```python
from build123d import *

# Parameters (mm, degrees)
CUT_EXTRUDE1_DEPTH = 4.7625
SKETCH6_R          = 2.749630657
CUT_EXTRUDE4_DEPTH = 4.7625
CUT_EXTRUDE4_DRAFT = -45


with BuildPart() as part:
    # Sketch4 → Revolve1 (revolve)
    with BuildSketch(Plane(origin=(0, 0, 0), x_dir=(0, 0, -1), z_dir=(1, 0, 0))):
        Polygon((-28.575, 7.14375), (-34.210625, 7.14375), (-34.925, 6.429375), (-34.925, 0), (22.225, 0), (22.225, 4.500033333), (21.962533333, 4.7625), (-26.2128, 4.7625), (-26.450925, 4.524375), (-28.336875, 4.524375), (-28.575, 4.7625), align=None)
    revolve(axis=Axis((0, 0, 34.925), (0, 0, -1)))

    # Sketch5 → Cut-Extrude1 (cut)
    with BuildSketch(Plane.XY.offset(34.925)):
        Polygon((2.38125, 1.374815329), (0, 2.749630657), (-2.38125, 1.374815329), (-2.38125, -1.374815329), (0, -2.749630657), (2.38125, -1.374815329), align=None)
    extrude(amount=-CUT_EXTRUDE1_DEPTH, mode=Mode.SUBTRACT)


with BuildPart() as cut_extrude4_tool:
    # Sketch6 → Cut-Extrude4 (with draft: the straight prism first)
    with BuildSketch(Plane.XY.offset(34.925)):
        Circle(SKETCH6_R)
    extrude(amount=-CUT_EXTRUDE4_DEPTH)
    # Cut-Extrude4: the draft: its side faces are tilted about the plane it starts from
    cut_extrude4_sides = [cut_extrude4_tool.faces().sort_by_distance(p)[0] for p in [
        (-2.749630657, 0, 32.54375),
    ]]
    draft(cut_extrude4_sides, Plane.XY.offset(34.925), CUT_EXTRUDE4_DRAFT)


with BuildPart() as part_1:
    add(part.part)

    # Cut-Extrude4: cut by cut_extrude4_tool
    add(cut_extrude4_tool.part, mode=Mode.SUBTRACT)

    # Sketch7 → Revolve2 (revolve)
    with BuildSketch(Plane(origin=(0, 0, 0), x_dir=(0, 0, -1), z_dir=(1, 0, 0))):
        Polygon((22.225, 3.9751), (33.866666667, 3.9751), (34.925, 2.916766667), (34.925, 0), (22.225, 0), align=None)
    revolve(axis=Axis((0, 0, -34.925), (0, 0, 1)))

    # Sketch10 → Cut-Revolve1 (revolve, cut)
    with BuildSketch(Plane(origin=(0, 0, 0), x_dir=(0, 0, -1), z_dir=(1, 0, 0))):
        with BuildLine():
            Line((23.1902, 3.0099), (25.0444, 3.0099))
            Line((25.0444, 3.0099), (26.797, 4.7625))
            Line((26.797, 4.7625), (22.225, 4.7625))
            Line((22.225, 4.7625), (22.225, 3.9751))
            ThreePointArc((22.225, 3.9751), (22.507700535, 3.292600535), (23.1902, 3.0099))
        make_face()
    revolve(axis=Axis((0, 0, -34.925), (0, 0, 1)), mode=Mode.SUBTRACT)


solid = part_1.part
```
Work out the finished part from the listing and answer in its coordinate system (mm). A direction names the side the tool comes from. Give positions to 0.01 mm unless a question says otherwise; leave off trailing zeros. Write each loop counter-clockwise with the first axis right and the second up, starting at its lowest first coordinate (ties: lowest second). Pieces come first, ordered by that corner, then holes.
(1) The part is cut by section A-A on z = -5.5. Write down the section's boundary in (x, y) (1 decimal), plus the area to 3 significant figures.
Final values:
outline: circle Ø9.5 at (0, 0)
area: 71.3 mm2
(2) Flat-ended cylindrical pins translate along their axes: pin 1 Ø3 at (x, z) = (-5.5, 23.5) entering from +Y; pin 2 Ø4 at (x, z) = (1.5, 16.5) entering from +Y; pin 3 Ø6 at (x, y) = (5, 4) entering from -Z. Find the tip coordinate at first contact, or state that the pin passes through.
Final values:
pin 1: stops at y = 2.58
pin 2: stops at y = 4.76
pin 3: stops at z = -34.44
(3) The mould has two halves that part along X. Classify faces 1 (the cylindrical face through (-2.9, -3.78, 2.46)), 2 (the flat face through (0, 3, 34.925)), 3 (the conical face through (1.27, -2.23, 34.74)), 4 (the flat face through (-1.174, 2.072, 32.577)): pulls with the +X half, pulls with the -X half, needs draft (parallel to the pull), parting line crosses it, or undercut.
Final values:
face 1: parting line crosses it
face 2: needs draft
face 3: undercut
face 4: undercut
(4) Straight lines are drawn through the part: line 1 (Z direction, x = 4.25, y = 2.5) (3 decimals); line 2 (Z direction, x = -3.25, y = -3) (3 decimals); line 3 (X direction, y = 1, z = -15). For each, find the intervals that lie inside material, in ascending order.
Final values:
line 1: z = 28.575 to 34.925
line 2: z = -22.225 to 34.925
line 3: x = -4.66 to 4.66
(5) Which of the six approach directions +Z, -Z, +X, -X, +Y, -Y give full straight-line access (tool end or side, diameter ignored) to faces 5 (the cylindrical face through (0.314, -7.137, 31.432)), 6 (the flat face through (-3, -3, -22.225)), 7 (the flat face through (0, 0, 30.162)), 8 (the cylindrical face through (-2.753, -3.59, 27.407))?
Final values:
face 5: +Z, -Z
face 6: -Z
face 7: +Z
face 8: none
